```python
from build123d import *

# Parameters (mm, degrees)
BOSS_EXTRUDE1_DEPTH                             = 70
SKETCH2_W                                       = 100.495668723
SKETCH2_H                                       = 40
CUT_EXTRUDE1_DEPTH                              = 91.277350426
SKETCH3_R                                       = 3.75
CUT_EXTRUDE2_DEPTH                              = 10
SKETCH4_R                                       = 3.75
CUT_EXTRUDE3_DEPTH                              = 10
SKETCH5_R                                       = 3.75
CUT_EXTRUDE4_DEPTH                              = 110.201648339
CSK_FOR_M2_FLAT_HEAD_MACHINE_SCREW1_D           = 2.4
CSK_FOR_M2_FLAT_HEAD_MACHINE_SCREW1_CSINK_D     = 4.4
CSK_FOR_M2_FLAT_HEAD_MACHINE_SCREW1_CSINK_ANGLE = 90


with BuildPart() as part:
    # Sketch1 → Boss-Extrude1 (new body)
    with BuildSketch(Plane.XY):
        with BuildLine():
            Line((-35, 10), (-35, 25))
            Line((-35, 25), (-45, 25))
            Line((-45, 25), (-45, -25))
            Line((-45, -25), (-35, -25))
            Line((-35, -25), (-35, -10))
            Line((-35, -10), (35, -10))
            ThreePointArc((35, -10), (45, 0), (35, 10))
            Line((35, 10), (-35, 10))
        make_face()
    extrude(amount=-BOSS_EXTRUDE1_DEPTH)

    # Sketch2 → Cut-Extrude1 (cut, through all)
    with BuildSketch(Plane(origin=(0, 10, 0), x_dir=(1, 0, 0), z_dir=(0, 1, 0))):
        with Locations((15.247834362, 35)):
            Rectangle(SKETCH2_W, SKETCH2_H)
    extrude(amount=-CUT_EXTRUDE1_DEPTH, mode=Mode.SUBTRACT)

    # Sketch3 → Cut-Extrude2 (cut)
    with BuildSketch(Plane.XY.offset(-55)):
        with Locations((35, 0)):
            Circle(SKETCH3_R)
    extrude(amount=-CUT_EXTRUDE2_DEPTH, mode=Mode.SUBTRACT)

    # Sketch4 → Cut-Extrude3 (cut)
    with BuildSketch(Plane(origin=(0, 0, -15), x_dir=(-1, 0, 0), z_dir=(0, 0, -1))):
        with Locations((-33.885516641, 0)):
            Circle(SKETCH4_R)
    extrude(amount=-CUT_EXTRUDE3_DEPTH, mode=Mode.SUBTRACT)

    # Sketch5 → Cut-Extrude4 (cut, through all)
    with BuildSketch(Plane(origin=(-35, 0, 0), x_dir=(0, 0, -1), z_dir=(1, 0, 0))):
        with Locations((35, 0)):
            Circle(SKETCH5_R)
    extrude(amount=-CUT_EXTRUDE4_DEPTH, mode=Mode.SUBTRACT)

    # CSK for M2 Flat Head Machine Screw1 (through all)
    with Locations(Plane.ZY.offset(45)):
        with Locations((-50, 15), (-20, 15), (-20, -15), (-50, -15)):
            CounterSinkHole(CSK_FOR_M2_FLAT_HEAD_MACHINE_SCREW1_D / 2, CSK_FOR_M2_FLAT_HEAD_MACHINE_SCREW1_CSINK_D / 2, counter_sink_angle=CSK_FOR_M2_FLAT_HEAD_MACHINE_SCREW1_CSINK_ANGLE)


solid = part.part
```
The listing builds one solid part. Answer for the finished solid, in the listing's coordinates (mm). A direction names the side the tool comes from. Round coordinates to 2 decimals unless told otherwise and drop trailing zeros. Loops run counter-clockwise (first coordinate to the right, second up) from the corner with the lowest first, then second, coordinate; pieces in that order, holes last.
Q1. Section D-D, the plane y = 15 is taken. Determine the outline of the cut face in (x, z), then the cut area to 3 significant figures.
Q2. Section C-C, the plane y = 0 is taken. Determine the outline of the cut face in (x, z), then the cut area to 4 significant figures.
Q3. Section B-B, the plane x = -34 is taken. Determine the outline of the cut face in (y, z).
Q4. Which of the six approach directions +Z, -Z, +X, -X, +Y, -Y give full straight-line access (tool end or side, diameter ignored) to faces 5 (the face through (35, 0, -65)), 6 (the face through (-40, -25, -35)), 7 (the face through (4, 0, -15)), 8 (the face through (0, 10, -62)), 9 (the face through (0, -10, -7))?
Q5. Section A-A, the plane z = -35 is taken. Determine the outline of the cut face in (x, y).
Q6. Find the intervals of material crossed by line 1 (Z direction, x = -37, y = 15); line 2 (Z direction, x = 17, y = 6.5); line 3 (Y direction, x = 35, z = -61), in increasing order.
Q7. Given pin 1 Ø12 at (x, z) = (6, -63) entering from -Y; pin 2 Ø3 at (y, z) = (7, -42.5) entering from +X; pin 3 Ø12 at (x, z) = (4, -62.5) entering from +Y, each flat-ended and moving along its own axis, determine where each tip first touches the part or whether it passes through.
Q8. For a pull along X with two mould halves and no side action, classify faces 1 (the face through (-40, 25, -35)), 2 (the face through (-35, -6, -35)), 3 (the face through (30.3, 1.1, -10.1)), 4 (the face through (34, 0, -5)) as released by +X, released by -X, zero draft, split by the parting line, or undercut.
Completed:
1. outline: (-45, -70) - (-35, -70) - (-35, -51.2) - (-44, -51.2) - (-45, -52.2) - close; (-45, -47.8) - (-44, -48.8) - (-35, -48.8) - (-35, -21.2) - (-44, -21.2) - (-45, -22.2) - close; (-45, -17.8) - (-44, -18.8) - (-35, -18.8) - (-35, 0) - (-45, 0) - close
1. area: 650 mm2
2. outline: (-45, -70) - (45, -70) - (45, -55) - (38.75, -55) - (38.75, -65) - (31.25, -65) - (31.25, -55) - (-35, -55) - (-35, -38.75) - (-45, -38.75) - close; (-45, -31.25) - (-35, -31.25) - (-35, -15) - (30.14, -15) - (30.14, -5) - (37.64, -5) - (37.64, -15) - (45, -15) - (45, 0) - (-45, 0) - close
2. area: 2,875 mm2
3. outline: (-10, -70) - (10, -70) - (10, -55) - (-10, -55) - close; (-10, -15) - (10, -15) - (10, 0) - (-10, 0) - close
4. face 5: none
4. face 6: +Z, -Z, +X, -X, -Y
4. face 7: +X, +Y, -Y
4. face 8: +Z, -Z, +X, +Y
4. face 9: +Z, -Z, +X, -Y
5. outline: (-45, -25) - (-35, -25) - (-35, -3.75) - (-45, -3.75) - close; (-45, 3.75) - (-35, 3.75) - (-35, 25) - (-45, 25) - close
6. line 1: z = -70 to -51.2, -48.8 to -21.2, -18.8 to 0
6. line 2: z = -70 to -55, -15 to 0
6. line 3: y = -10 to -3.75, 3.75 to 10
7. pin 1: stops at y = -10
7. pin 2: stops at x = -35
7. pin 3: stops at y = 10
8. face 1: zero draft
8. face 2: released by +X
8. face 3: undercut
8. face 4: undercut
